Model file for the job. Use its own axes, mm. Face numbers are marked on the shaded views. A direction names the side the tool comes from. Round coordinates to 2 decimals unless told otherwise and drop trailing zeros. Order: outer loops, then holes, each group sorted by start corner. A loop starts at its lowest first (then second) coordinate and runs counter-clockwise, first axis right, second up. Notation, with made-up numbers: (30.25, -13.5) - (65.25, -13.5) arc R25 cw to (65.25, 4.5) - close; hole circle Ø2 at (43.25, 12.25). An arc over 180 degrees is marked (long way). Answer as CSV lines item,"result". Start each with the question number.
1. Band-saw the part on C-C on x = -12. List the corners of the cut face in (y, z), then the cut area to 3 significant figures.
2. Band-saw the part on B-B on y = 12. List the corners of the cut face in (x, z).
3. Pull direction X, two halves, no side cores. Call the marked faces 3, 4 and 5: released by +X, released by -X, zero draft, split by the parting line, or undercut.
4. Pin check, flat tip, straight feed: pin 1 Ø6.5 at (x, z) = (0, 10) entering from -Y. Stop position of the tip, or through.
5. 3-axis set-ups, long thin cutter, end or side, ignore diameter. For the marked faces 1 and 2: which of +Z, -Z, +X, -X, +Y, -Y reach the whole face in a straight line?
6. Band-saw the part on D-D on x = 0. List the corners of the cut face in (y, z), then the cut area to 3 significant figures.
7. Band-saw the part on A-A on z = 10. List the corners of the cut face in (x, y).
8. Wall check: line 1 along X through (y, z) = (-8, 54); line 2 along Y through (x, z) = (-19, 55.5); line 3 along Z through (x, y) = (0, -33.1). Give the ranges that are in metal, low to high. Write a range as [from, to].
```python
from build123d import *

# Parameters (mm, degrees)
F0_W     = 60
F0_H     = 70
F0_W_2   = 50
F0_H_2   = 60
F1_DEPTH = 60
F2_F1_R  = 2
F2_F2_R  = 2
F4_R     = 3.5
F5_DEPTH = 70


with BuildPart() as f1:
    # F0 (on Top) → F1 (new body)
    with BuildSketch(Plane.XY):
        Rectangle(F0_W, F0_H)
        Rectangle(F0_W_2, F0_H_2, mode=Mode.SUBTRACT)
    extrude(amount=F1_DEPTH)

    # F2: fillet of radius 2 on 16 edges, made by hand

    # F2_f1
    f2_f1_edges = [f1.edges().sort_by_distance(p)[0] for p in [
        (-25, -30, 30),
        (25, -30, 30),
        (25, 30, 30),
        (-25, 30, 30),
    ]]
    fillet(f2_f1_edges, radius=F2_F1_R)

    # F2_f2
    f2_f2_edges = [f1.edges().sort_by_distance(p)[0] for p in [
        (-30, 35, 30),
        (0, 35, 60),
        (30, 35, 30),
        (0, 35, 0),
        (30, -35, 30),
        (0, -35, 60),
        (-30, -35, 30),
        (0, -35, 0),
        (0, -30, 60),
        (0, -30, 0),
        (0, 30, 60),
        (0, 30, 0),
        (-24.4142135624, 29.4142135624, 0),
        (24.4142135624, 29.4142135624, 0),
        (-24.4142135624, 29.4142135624, 60),
        (24.4142135624, 29.4142135624, 60),
        (24.4142135624, -29.4142135624, 0),
        (-24.4142135624, -29.4142135624, 0),
        (24.4142135624, -29.4142135624, 60),
        (-24.4142135624, -29.4142135624, 60),
    ]]
    fillet(f2_f2_edges, radius=F2_F2_R)

    # F4 (on face) → F5 (cut)
    with BuildSketch(Plane(origin=(0, 35, 0), x_dir=(-1, 0, 0), z_dir=(0, 1, 0))):
        with Locations((0, 10)):
            Circle(F4_R)
    extrude(amount=-F5_DEPTH, mode=Mode.SUBTRACT)


solid = f1.part
```
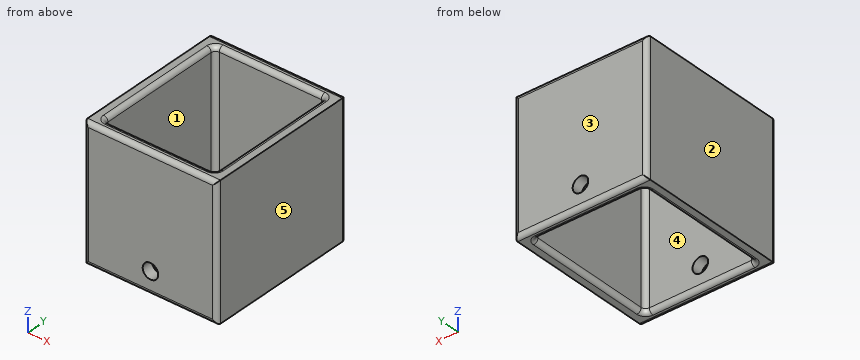
Reply:
1,outline,"(-35, 2) arc R2 ccw to (-33, 0) - (-32, 0) arc R2 ccw to (-30, 2) - (-30, 58) arc R2 ccw to (-32, 60) - (-33, 60) arc R2 ccw to (-35, 58) - close; (30, 2) arc R2 ccw to (32, 0) - (33, 0) arc R2 ccw to (35, 2) - (35, 58) arc R2 ccw to (33, 60) - (32, 60) arc R2 ccw to (30, 58) - close"
1,area,"593 mm2"
2,outline,"(-30, 0) - (-27, 0) arc R2 ccw to (-25, 2) - (-25, 58) arc R2 ccw to (-27, 60) - (-30, 60) - close; (25, 2) arc R2 ccw to (27, 0) - (30, 0) - (30, 60) - (27, 60) arc R2 ccw to (25, 58) - close"
3,face 3,"zero draft"
3,face 4,"undercut"
3,face 5,"released by +X"
4,pin 1,"passes through"
5,face 1,"+Z, -Z"
5,face 2,"+Z, -Z, -X, +Y, -Y"
6,outline,"(-35, 2) arc R2 ccw to (-33, 0) - (-32, 0) arc R2 ccw to (-30, 2) - (-30, 6.5) - (-35, 6.5) - close; (-35, 13.5) - (-30, 13.5) - (-30, 58) arc R2 ccw to (-32, 60) - (-33, 60) arc R2 ccw to (-35, 58) - close; (30, 2) arc R2 ccw to (32, 0) - (33, 0) arc R2 ccw to (35, 2) - (35, 6.5) - (30, 6.5) - close; (30, 13.5) - (35, 13.5) - (35, 58) arc R2 ccw to (33, 60) - (32, 60) arc R2 ccw to (30, 58) - close"
6,area,"523 mm2"
7,outline,"(-30, -33) arc R2 ccw to (-28, -35) - (-3.5, -35) - (-3.5, -30) - (-23, -30) arc R2 cw to (-25, -28) - (-25, 28) arc R2 cw to (-23, 30) - (-3.5, 30) - (-3.5, 35) - (-28, 35) arc R2 ccw to (-30, 33) - close; (3.5, -35) - (28, -35) arc R2 ccw to (30, -33) - (30, 33) arc R2 ccw to (28, 35) - (3.5, 35) - (3.5, 30) - (23, 30) arc R2 cw to (25, 28) - (25, -28) arc R2 cw to (23, -30) - (3.5, -30) - close"
8,line 1,"x = [-30, -25], [25, 30]"
8,line 2,"y = [-35, -30], [30, 35]"
8,line 3,"z = [0, 6.5], [13.5, 60]"
